Autodesk Inventor part; units mm, degrees
ref_plane "Plano inicial" through (0, 0, 0) normal (0, 0, 1) x (1, 0, 0)
ref_plane "Plano final" through (0, 0, 490) normal (0, 0, 1) x (1, 0, 0)
ref_plane "Plano de trabalho4" through (0, -25, 0) normal (0, 0.7071, -0.7071) x (1, 0, 0)
ref_plane "Plano inicial" through (0, 0, 0) normal (0, 0, 1) x (1, 0, 0)
ref_plane "Plano final" through (0, 0, 490) normal (0, 0, 1) x (1, 0, 0)
sketch "Esboço" plane through (0, 0, 0) normal (0, 0, 1) x (1, 0, 0)
  line L0 (-15, -21) -> (-15, 21)
  line L1 (-11, 25) -> (11, 25)
  line L2 (15, 21) -> (15, -21)
  line L3 (11, -25) -> (-11, -25)
  arc A0 (-15, -21) -> (-11, -25) centre (-11, -21) ccw
  arc A1 (15, 21) -> (11, 25) centre (11, 21) ccw
  arc A2 (-11, 25) -> (-15, 21) centre (-11, 21) ccw
  arc A3 (11, -25) -> (15, -21) centre (11, -21) ccw
  arc A4 (-11, 23) -> (-13, 21) centre (-11, 21) ccw
  line L4 (-11, 23) -> (11, 23)
  arc A5 (13, 21) -> (11, 23) centre (11, 21) ccw
  line L5 (13, 21) -> (13, -21)
  arc A6 (11, -23) -> (13, -21) centre (11, -21) ccw
  line L6 (11, -23) -> (-11, -23)
  arc A7 (-13, -21) -> (-11, -23) centre (-11, -21) ccw
  line L7 (-13, -21) -> (-13, 21)
  line L8 (0, 36.1598) -> (0, -36.1598) construction
  line L9 (-22.1598, 0) -> (22.1598, 0) construction
  dimension "d7" = 4
  dimension "d9" = 30
  dimension "d11" = 50
  dimension "d12" = 2
  dimension "d15" = 15
  dimension "d16" = 25
extrude "Corpo" add sketch "Esboço" along normal up to surface (490 mm away) from surface at 0
sketch "Sketch3" plane through (0, 0, 0) normal (0, 0, 1) x (1, 0, 0)
  line L0 (0, 0) -> (10, 0)
ref_plane "Work Plane3" through (0, 0, 0) normal (0, -1, 0) x (1, 0, 0)
sketch "Sketch4" plane through (0, 0, 0) normal (0, -1, 0) x (1, 0, 0)
  line L0 (-2, 0) -> (12, 0)
  line L1 (-2, 490) -> (12, 490)
  dimension "d18" = 490
ref_plane "Plano de trabalho4" through (0, -25, 0) normal (0, 0.7071, -0.7071) x (1, 0, 0)
split "Dividir1" plane through (0, -25, 0) removes the side toward (0, 0.7071, -0.7071)
equation "\"d7\" = G_IR"
equation "\"d9\" = G_W"
equation "\"d11\" = G_H"
equation "\"d12\" = G_T"
equation "\"d15\" = 0.5 * d9"
equation "\"d16\" = 0.5 * d11"
equation "\"d3\" = G_L"
equation "\"G_W\" = 30"
equation "\"G_H\" = 50"
equation "\"G_T\" = 2"
equation "\"G_IR\" = 4"
equation "\"G_L\" = d18"
equation "\"G_OFFSET_START\" = 0"
equation "\"G_OFFSET_END\" = 0"
properties part number "ISO 4019 - 50x30x2 - 490" material "Aço, suave"
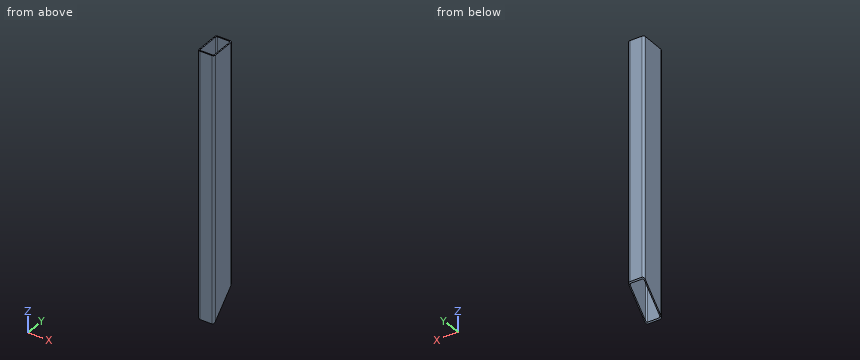
Part model, mm, in its own coordinate system. Give positions to 0.01 mm unless a question says otherwise; leave off trailing zeros. Write each loop counter-clockwise with the first axis right and the second up, starting at its lowest first coordinate (ties: lowest second). Pieces come first, ordered by that corner, then holes. Notation, with made-up numbers: (3.25, 14) -> (54.25, 14) arc R5 cw to (54.25, 20) -> close; hole circle Ø6 at (41, 73.25). An arc over 180 degrees is marked (long way). Put each result on its own line as item: value. Start each with the question number.
Item 1: Cut at B-B (z = 325). List the corners of the cut face in (x, y).
Item 2: Cut at A-A (y = 12.5). List the corners of the cut face in (x, z).
Item 3: Cut at C-C (x = -0.25). List the corners of the cut face in (y, z).
Item 4: Wall check: L1, parallel to X at y = -9, z = 403; L2, parallel to Y at x = -7.5, z = 282; L3, parallel to Y at x = -12, z = 428.5. Give the ranges that are in metal, low to high. Write a range as [from, to].
Answer list:
1. outline: (-15, -21) arc R4 ccw to (-11, -25) -> (11, -25) arc R4 ccw to (15, -21) -> (15, 21) arc R4 ccw to (11, 25) -> (-11, 25) arc R4 ccw to (-15, 21) -> close; hole (-13, -21) arc R2 ccw to (-11, -23) -> (11, -23) arc R2 ccw to (13, -21) -> (13, 21) arc R2 ccw to (11, 23) -> (-11, 23) arc R2 ccw to (-13, 21) -> close
2. outline: (-15, 37.5) -> (-13, 37.5) -> (-13, 490) -> (-15, 490) -> close; (13, 37.5) -> (15, 37.5) -> (15, 490) -> (13, 490) -> close
3. outline: (-25, 0) -> (-23, 2) -> (-23, 490) -> (-25, 490) -> close; (23, 48) -> (25, 50) -> (25, 490) -> (23, 490) -> close
4. L1: x = [-15, -13], [13, 15]
4. L2: y = [-25, -23], [23, 25]
4. L3: y = [-24.87, -22.73], [22.73, 24.87]
